For this review, take the finished solid that the model builds, in its own axes (mm). Give positions to 0.01 mm unless a question says otherwise; leave off trailing zeros. Write each loop counter-clockwise with the first axis right and the second up, starting at its lowest first coordinate (ties: lowest second). Pieces come first, ordered by that corner, then holes. Notation, with made-up numbers: (-5, 42) -> (15, 42) arc R25 cw to (15, 67) -> close; hole circle Ø1 at (46, 34.5). An arc over 180 degrees is marked (long way). Answer as CSV lines item,"result".
```python
from build123d import *

# Parameters (mm, degrees)
SKETCH1_W           = 430
SKETCH1_H           = 76.2
SKETCH1_R           = 4.5
SKETCH1_R_2         = 3.25
BOSS_EXTRUDE1_DEPTH = 6.35
CHAMFER1_SIZE       = 4.5


with BuildPart() as part:
    # Sketch1 → Boss-Extrude1 (new body)
    with BuildSketch(Plane.XY):
        with Locations((215, 38.1)):
            Rectangle(SKETCH1_W, SKETCH1_H)
        with Locations((9, 58.1)):
            Circle(SKETCH1_R, mode=Mode.SUBTRACT)
        with Locations(Location((9, 18.1, 0), (0, 0, 180))):
            Circle(SKETCH1_R, mode=Mode.SUBTRACT)
        with Locations((421, 18.1)):
            Circle(SKETCH1_R, mode=Mode.SUBTRACT)
        with Locations(Location((421, 58.1, 0), (0, 0, 180))):
            Circle(SKETCH1_R, mode=Mode.SUBTRACT)
        with Locations((33.75, 38.1)):
            Circle(SKETCH1_R_2, mode=Mode.SUBTRACT)
        with Locations((363.75, 38.1)):
            Circle(SKETCH1_R_2, mode=Mode.SUBTRACT)
    extrude(amount=BOSS_EXTRUDE1_DEPTH)

    # Chamfer1
    chamfer1_edges = [part.edges().sort_by_distance(p)[0] for p in [
        (4.5, 58.1, 0),
        (13.5, 18.1, 0),
        (416.5, 18.1, 0),
        (425.5, 58.1, 0),
    ]]
    chamfer(chamfer1_edges, length=CHAMFER1_SIZE - 0.0001)  # a hair under: the kernel refuses the full size


solid = part.part
```
Q1. Draft analysis for pull direction X (two halves, no side actions). For faces 1 (the cylindrical face through (11.08, 54.11, 5.41)), 2 (the flat face through (212, 39, 0)), 3 (the conical face through (426, 58, 4)), state which applies: released by +X, released by -X, zero draft, split by the parting line, or undercut.
Answer block:
face 1,"undercut"
face 2,"zero draft"
face 3,"undercut"
Q2. Clearance check with flat-ended pins moving along their axes: pin 1 (4 mm diameter, centred on x = 363.75, y = 38.1, fed in from +Z); pin 2 (10.5 mm diameter, centred on x = 9, y = 18.1, fed in from -Z); pin 3 (14.5 mm diameter, centred on x = 9, y = 58.1, fed in from -Z); pin 4 (11.5 mm diameter, centred on x = 421, y = 18.1, fed in from -Z). State where each tip first meets the part, or that it passes through.
Answer block:
pin 1,"passes through"
pin 2,"stops at z = 3.75"
pin 3,"stops at z = 1.75"
pin 4,"stops at z = 3.25"
Q3. To check wall thickness, follow probe 1 along Y at (x, z) = (421, 5.85); probe 2 along Y at (x, z) = (33.75, 1.5); probe 3 along X at (y, z) = (64, 1.75). State the ranges of each line that lie inside material, in increasing order. Write a range as [from, to].
Answer block:
probe 1,"y = [0, 13.6], [22.6, 53.6], [62.6, 76.2]"
probe 2,"y = [0, 34.85], [41.35, 76.2]"
probe 3,"x = [0, 4.79], [13.21, 416.79], [425.21, 430]"
Q4. Add section B-B (x = 421). Write out the cut boundary in (y, z), plus the area to 3 significant figures.
Answer block:
outline,"(0, 0) -> (9.1, 0) -> (13.6, 4.5) -> (13.6, 6.35) -> (0, 6.35) -> close; (22.6, 4.5) -> (27.1, 0) -> (49.1, 0) -> (53.6, 4.5) -> (53.6, 6.35) -> (22.6, 6.35) -> close; (62.6, 4.5) -> (67.1, 0) -> (76.2, 0) -> (76.2, 6.35) -> (62.6, 6.35) -> close"
area,"329 mm2"
Q5. Add section A-A (y = 18.1). State how many separate pieces and enclosed holes the cut face has, plus the area to 3 significant figures.
Answer block:
separate pieces,"3"
enclosed holes,"0"
area,"2,580 mm2"
Q6. Add section C-C (z = 1.75). Write out the cut boundary in (x, y), plus the area to 3 significant figures.
Answer block:
outline,"(0, 0) -> (430, 0) -> (430, 76.2) -> (0, 76.2) -> close; hole circle Ø14.5 at (9, 18.1); hole circle Ø14.5 at (9, 58.1); hole circle Ø6.5 at (33.75, 38.1); hole circle Ø6.5 at (363.75, 38.1); hole circle Ø14.5 at (421, 18.1); hole circle Ø14.5 at (421, 58.1)"
area,"32,000 mm2"
